Autodesk Inventor part; units mm, degrees
ref_plane "Start plane" through (0, 0, -17.5) normal (0, 0, 1) x (1, 0, 0)
ref_plane "End plane" through (0, 0, 797.5) normal (0, 0, 1) x (1, 0, 0)
ref_plane "Work Plane4" through (107.5, 0, -17.5) normal (0, 0, -1) x (-1, 0, 0)
ref_plane "Start plane" through (0, 0, -17.5) normal (0, 0, 1) x (1, 0, 0)
ref_plane "End plane" through (0, 0, 797.5) normal (0, 0, 1) x (1, 0, 0)
sketch "Sketch" plane through (0, 0, 0) normal (0, 0, 1) x (1, 0, 0)
  line L0 (-17.5, -12.5) -> (-17.5, 12.5)
  line L1 (-12.5, 17.5) -> (12.5, 17.5)
  line L2 (17.5, 12.5) -> (17.5, -12.5)
  line L3 (12.5, -17.5) -> (-12.5, -17.5)
  arc A0 (-17.5, -12.5) -> (-12.5, -17.5) centre (-12.5, -12.5) ccw
  arc A1 (-12.5, 17.5) -> (-17.5, 12.5) centre (-12.5, 12.5) ccw
  arc A2 (17.5, 12.5) -> (12.5, 17.5) centre (12.5, 12.5) ccw
  arc A3 (12.5, -17.5) -> (17.5, -12.5) centre (12.5, -12.5) ccw
  arc A4 (-12.5, 15) -> (-15, 12.5) centre (-12.5, 12.5) ccw
  line L4 (-12.5, 15) -> (12.5, 15)
  arc A5 (15, 12.5) -> (12.5, 15) centre (12.5, 12.5) ccw
  line L5 (15, 12.5) -> (15, -12.5)
  arc A6 (12.5, -15) -> (15, -12.5) centre (12.5, -12.5) ccw
  line L6 (12.5, -15) -> (-12.5, -15)
  arc A7 (-15, -12.5) -> (-12.5, -15) centre (-12.5, -12.5) ccw
  line L7 (-15, -12.5) -> (-15, 12.5)
  line L8 (0, 25.9497) -> (0, -25.9497) construction
  line L9 (-25.9497, 0) -> (25.9497, 0) construction
  dimension "d7" = 5
  dimension "d10" = 35
  dimension "d11" = 35
  dimension "d12" = 2.5
  dimension "d15" = 17.5
  dimension "d16" = 17.5
extrude "Body" add sketch "Sketch" along normal up to surface (815 mm away) from surface at -17.5
sketch "Sketch3" plane through (0, 0, 0) normal (0, 0, 1) x (1, 0, 0)
  line L0 (0, 0) -> (10, 0)
ref_plane "Work Plane3" through (0, 0, 0) normal (0, -1, 0) x (1, 0, 0)
sketch "Sketch4" plane through (0, 0, 0) normal (0, -1, 0) x (1, 0, 0)
  line L0 (-2, -17.5) -> (12, -17.5)
  line L1 (-2, 797.5) -> (12, 797.5)
  dimension "d18" = 815
ref_plane "Work Plane4" through (107.5, 0, -17.5) normal (0, 0, -1) x (-1, 0, 0)
split "Split1" plane through (107.5, 0, -17.5) removes the side toward (0, 0, -1)
ref_plane "Work Plane5" through (17.5, 0, 797.5) normal (0, 0, 1) x (1, 0, 0)
split "Split2" plane through (17.5, 0, 797.5) removes the side toward (0, 0, 1)
ref_plane "Work Plane6" through (0, 17.5, -17.5) normal (0, -0.7071, -0.7071) x (1, 0, 0)
split "Split3" plane through (0, 17.5, -17.5) removes the side toward (0, -0.7071, -0.7071)
ref_plane "Work Plane14" through (0, 17.5, 797.5) normal (0, -0.7071, 0.7071) x (1, 0, 0)
split "Split5" plane through (0, 17.5, 797.5) removes the side toward (0, -0.7071, 0.7071)
ref_plane "Work Plane17" through (0, 10, 190) normal (0, -1, 0) x (0, 0, -1)
ref_plane "Work Plane18" through (0, -490, 190) normal (0, -1, 0) x (0, 0, -1)
ref_plane "Work Plane19" through (0, -240, 190) normal (0, -1, 0) x (0, 0, -1)
ref_plane "Work Plane20" through (0, 0, 390) normal (0, -1, 0) x (0, 0, -1)
ref_plane "Work Plane21" through (0, -480, 390) normal (0, -1, 0) x (0, 0, -1)
ref_plane "Work Plane22" through (0, -240, 390) normal (0, -1, 0) x (0, 0, -1)
ref_plane "Work Plane23" through (0, 10, 590) normal (0, -1, 0) x (0, 0, -1)
ref_plane "Work Plane24" through (0, -490, 590) normal (0, -1, 0) x (0, 0, -1)
ref_plane "Work Plane25" through (0, -240, 590) normal (0, -1, 0) x (0, 0, -1)
sketch "Sketch17" plane through (0, -240, 190) normal (0, -1, 0) x (0, 0, -1)
  arc A0 (-17.5, -12.5) -> (-12.5, -17.5) centre (-12.5, -12.5) ccw
  line L0 (-17.5, -12.5) -> (-17.5, 12.5)
  arc A1 (-12.5, 17.5) -> (-17.5, 12.5) centre (-12.5, 12.5) ccw
  line L1 (-12.5, 17.5) -> (12.5, 17.5)
  arc A2 (17.5, 12.5) -> (12.5, 17.5) centre (12.5, 12.5) ccw
  line L2 (17.5, 12.5) -> (17.5, -12.5)
  arc A3 (12.5, -17.5) -> (17.5, -12.5) centre (12.5, -12.5) ccw
  line L3 (12.5, -17.5) -> (-12.5, -17.5)
  arc A4 (-12.5, 15) -> (-15, 12.5) centre (-12.5, 12.5) ccw
  line L4 (-12.5, 15) -> (12.5, 15)
  arc A5 (15, 12.5) -> (12.5, 15) centre (12.5, 12.5) ccw
  line L5 (15, 12.5) -> (15, -12.5)
  arc A6 (12.5, -15) -> (15, -12.5) centre (12.5, -12.5) ccw
  line L6 (12.5, -15) -> (-12.5, -15)
  arc A7 (-15, -12.5) -> (-12.5, -15) centre (-12.5, -12.5) ccw
  line L7 (-15, -12.5) -> (-15, 12.5)
extrude "Extrusion14" cut sketch "Sketch17" along normal up to surface (500 mm away) from surface at -250 contours L0 A1 L1 A2 L2 A3 L3 A0 | L4 A5 L5 A6 L6 A7 L7 A4
sketch "Sketch18" plane through (0, -240, 390) normal (0, -1, 0) x (0, 0, -1)
  arc A0 (-17.5, -12.5) -> (-12.5, -17.5) centre (-12.5, -12.5) ccw
  line L0 (-17.5, -12.5) -> (-17.5, 12.5)
  arc A1 (-12.5, 17.5) -> (-17.5, 12.5) centre (-12.5, 12.5) ccw
  line L1 (-12.5, 17.5) -> (12.5, 17.5)
  arc A2 (17.5, 12.5) -> (12.5, 17.5) centre (12.5, 12.5) ccw
  line L2 (17.5, 12.5) -> (17.5, -12.5)
  arc A3 (12.5, -17.5) -> (17.5, -12.5) centre (12.5, -12.5) ccw
  line L3 (12.5, -17.5) -> (-12.5, -17.5)
  arc A4 (-12.5, 15) -> (-15, 12.5) centre (-12.5, 12.5) ccw
  line L4 (-12.5, 15) -> (12.5, 15)
  arc A5 (15, 12.5) -> (12.5, 15) centre (12.5, 12.5) ccw
  line L5 (15, 12.5) -> (15, -12.5)
  arc A6 (12.5, -15) -> (15, -12.5) centre (12.5, -12.5) ccw
  line L6 (12.5, -15) -> (-12.5, -15)
  arc A7 (-15, -12.5) -> (-12.5, -15) centre (-12.5, -12.5) ccw
  line L7 (-15, -12.5) -> (-15, 12.5)
extrude "Extrusion15" cut sketch "Sketch18" along normal up to surface (480 mm away) from surface at -240 contours L0 A1 L1 A2 L2 A3 L3 A0 | L4 A5 L5 A6 L6 A7 L7 A4
sketch "Sketch19" plane through (0, -240, 590) normal (0, -1, 0) x (0, 0, -1)
  arc A0 (-17.5, -12.5) -> (-12.5, -17.5) centre (-12.5, -12.5) ccw
  line L0 (-17.5, -12.5) -> (-17.5, 12.5)
  arc A1 (-12.5, 17.5) -> (-17.5, 12.5) centre (-12.5, 12.5) ccw
  line L1 (-12.5, 17.5) -> (12.5, 17.5)
  arc A2 (17.5, 12.5) -> (12.5, 17.5) centre (12.5, 12.5) ccw
  line L2 (17.5, 12.5) -> (17.5, -12.5)
  arc A3 (12.5, -17.5) -> (17.5, -12.5) centre (12.5, -12.5) ccw
  line L3 (12.5, -17.5) -> (-12.5, -17.5)
  arc A4 (-12.5, 15) -> (-15, 12.5) centre (-12.5, 12.5) ccw
  line L4 (-12.5, 15) -> (12.5, 15)
  arc A5 (15, 12.5) -> (12.5, 15) centre (12.5, 12.5) ccw
  line L5 (15, 12.5) -> (15, -12.5)
  arc A6 (12.5, -15) -> (15, -12.5) centre (12.5, -12.5) ccw
  line L6 (12.5, -15) -> (-12.5, -15)
  arc A7 (-15, -12.5) -> (-12.5, -15) centre (-12.5, -12.5) ccw
  line L7 (-15, -12.5) -> (-15, 12.5)
extrude "Extrusion16" cut sketch "Sketch19" along normal up to surface (500 mm away) from surface at -250 contours L0 A1 L1 A2 L2 A3 L3 A0 | L4 A5 L5 A6 L6 A7 L7 A4
equation "\"d7\" = G_IR"
equation "\"d10\" = G_H"
equation "\"d11\" = G_W"
equation "\"d12\" = G_T"
equation "\"d15\" = 0.5 * d10"
equation "\"d16\" = 0.5 * d11"
equation "\"d3\" = G_L"
equation "\"G_W\" = 35"
equation "\"G_H\" = 35"
equation "\"G_T\" = 2.5"
equation "\"G_IR\" = 5"
equation "\"G_L\" = 835"
equation "\"G_OFFSET_START\" = 17.5"
equation "\"G_OFFSET_END\" = 17.5"
equation "\"d13\" = -G_OFFSET_START"
equation "\"d14\" = G_OFFSET_END + B_L"
properties part number "AS 1163 - C350L0 35x35x2.5 SHS - 835" material "Steel, Mild"
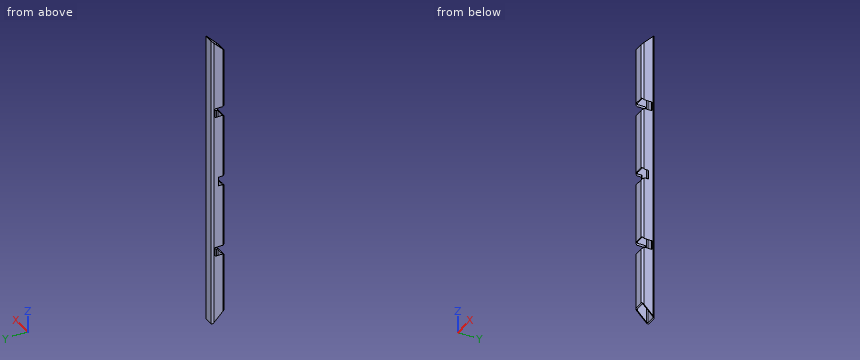
Input: part model. Units: mm. Frame: model coordinates. Give positions to 0.01 mm unless a question says otherwise; leave off trailing zeros. Order: outer loops, then holes, each group sorted by start corner. A loop starts at its lowest first (then second) coordinate and runs counter-clockwise, first axis right, second up. Notation, with made-up numbers: M 21,85 L 35,85 A30 ccw 35,118 Z; hole C 8,76.5 d7. An arc over 180 degrees is marked long. Return JSON: item names as keys, results as strings.
1) Contact query for flat-ended pins moving along their axis: pin 1 (12 mm diameter, centred on x = -1.5, z = 397, fed in from -Y); pin 2 (2 mm diameter, centred on x = 5.5, y = -17, fed in from +Z); pin 3 (0.8 mm diameter, centred on x = 0, y = -16.5, fed in from -Z); pin 4 (10 mm diameter, centred on x = -6, y = 4, fed in from -Z). Output: stop coordinate, or through.
Taken from the geometry:
{"pin 1": "stops at y = 15", "pin 2": "stops at z = 764", "pin 3": "stops at z = 16.1", "pin 4": "passes through"}
2) Section query A-A on y = -6.5. Count the separate pieces of the cut face and the enclosed holes in it, and give its area (3 significant figures).
Taken from the geometry:
{"separate pieces": "8", "enclosed holes": "0", "area": "3,370 mm2"}
3) Line query: L1, parallel to Y at x = -7.5, z = 361.5; L2, parallel to Z at x = -16, y = -6. Output: solid intervals per line, ascending. Write a range as [from, to].
Taken from the geometry:
{"L1": "y = [-17.5, -15], [15, 17.5]", "L2": "z = [6, 173.93], [206.07, 373.93], [406.07, 573.93], [606.07, 774]"}
4) Section query C-C on z = 108. Output: boundary loops of the cut face in (x, y).
Taken from the geometry:
{"outline": "M -17.5,-12.5 A5 ccw -12.5,-17.5 L 12.5,-17.5 A5 ccw 17.5,-12.5 L 17.5,12.5 A5 ccw 12.5,17.5 L -12.5,17.5 A5 ccw -17.5,12.5 Z; hole M -15,-12.5 A2.5 ccw -12.5,-15 L 12.5,-15 A2.5 ccw 15,-12.5 L 15,12.5 A2.5 ccw 12.5,15 L -12.5,15 A2.5 ccw -15,12.5 Z"}
5) Section query B-B on x = -5. Output: boundary loops of the cut face in (y, z), and give its area (3 significant figures).
Taken from the geometry:
{"outline": "M -17.5,17.5 L -15,15 L -15,172.5 L -17.5,172.5 Z; M -17.5,207.5 L -15,207.5 L -15,372.5 L -17.5,372.5 Z; M -17.5,407.5 L -15,407.5 L -15,572.5 L -17.5,572.5 Z; M -17.5,607.5 L -15,607.5 L -15,765 L -17.5,762.5 Z; M 15,-15 L 17.5,-17.5 L 17.5,797.5 L 15,795 Z", "area": "3,640 mm2"}
